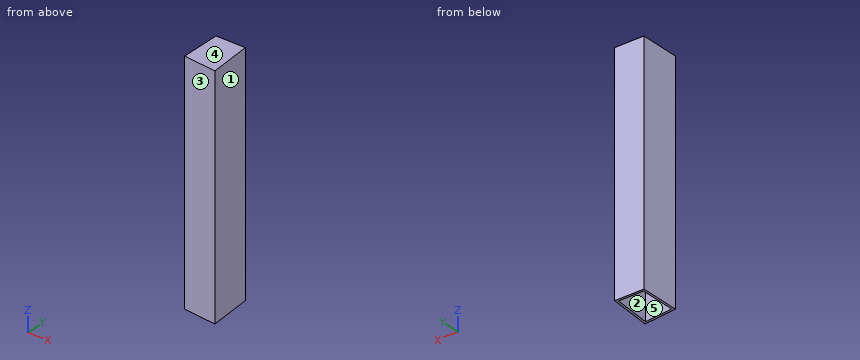
from build123d import *

# Parameters (mm, degrees)
F1_DEPTH = 25.4
F2_DEPTH = 233.172
F3_T     = -2.54


with BuildPart() as f1:
    # F0 (on Top) → F1 (new body)
    with BuildSketch(Plane.XY):
        Polygon((-96.244343, 37.27863), (-129.184976, 37.27863), (-129.184976, -7.511258), (-92.015967, -11.636118), align=None)
    extrude(amount=F1_DEPTH)

    # F0 (on Top) → F2 (join)
    with BuildSketch(Plane.XY):
        Polygon((-96.244343, 37.27863), (-129.184976, 37.27863), (-129.184976, -7.511258), (-92.015967, -11.636118), align=None)
    extrude(amount=-F2_DEPTH)

    # F3
    f3_openings = [f1.faces().sort_by_distance(p)[0] for p in [
        (-111.394879, 13.386796, -233.172),
    ]]
    offset(amount=F3_T, openings=f3_openings)


solid = f1.part
Check sheet for the modelled part. Datum: model origin and axes. Units: mm. Face numbers are marked on the shaded views. A direction names the side the tool comes from. Round coordinates to 2 decimals unless told otherwise and drop trailing zeros. Loops run counter-clockwise (first coordinate to the right, second up) from the corner with the lowest first, then second, coordinate; pieces in that order, holes last.
1. Sectioned sample at C-C on x = -111. Record the boundary of the cut face in (y, z), and give its area (3 significant figures).
2. Mould release check, pull along X, two halves, no side actions. Record for the marked faces 1, 2 and 3: released by +X, released by -X, zero draft, split by the parting line, or undercut.
3. Sectioned sample at A-A on z = -136. Record the boundary of the cut face in (x, y), and give its area (3 significant figures).
4. Set-up check for the marked faces 4 and 5: record each of +Z, -Z, +X, -X, +Y, -Y from which the full face is reachable in a straight line by a thin tool's end or side.
5. Gauge pin test, flat ends, axial feed: pin 1 Ø1.5 at (x, y) = (-122.5, 1) entering from -Z; pin 2 Ø12 at (y, z) = (13, -28) entering from +X; pin 3 Ø5 at (y, z) = (29.5, -94.5) entering from +X. Record the tip position at first contact, or that the pin passes through.
6. Scan lines: probe 1 along Z at (x, y) = (-107.5, 5.5); probe 2 along Y at (x, z) = (-99, -79.5); probe 3 along Y at (x, z) = (-120, -114). Record each from-to range of solid material in increasing order.
7. Sectioned sample at B-B on y = 22. Record the boundary of the cut face in (x, z), and give its area (3 significant figures).
Recorded:
1. outline: (-9.53, -233.17) - (-6.97, -233.17) - (-6.97, 22.86) - (34.74, 22.86) - (34.74, -233.17) - (37.28, -233.17) - (37.28, 25.4) - (-9.53, 25.4) - close
1. area: 1,420 mm2
2. face 1: released by +X
2. face 2: undercut
2. face 3: released by -X
3. outline: (-129.18, -7.51) - (-92.02, -11.64) - (-96.24, 37.28) - (-129.18, 37.28) - close; hole (-126.64, -5.24) - (-94.81, -8.77) - (-98.57, 34.74) - (-126.64, 34.74) - close
3. area: 391 mm2
4. face 4: +Z, +X, -X, +Y, -Y
4. face 5: -Z
5. pin 1: stops at z = 22.86
5. pin 2: stops at x = -93.63
5. pin 3: stops at x = -95.36
6. probe 1: z = 22.86 to 25.4
6. probe 2: y = -10.86 to -8.31, 34.74 to 37.28
6. probe 3: y = -8.53 to -5.97, 34.74 to 37.28
7. outline: (-129.18, -233.17) - (-126.64, -233.17) - (-126.64, 22.86) - (-97.47, 22.86) - (-97.47, -233.17) - (-94.92, -233.17) - (-94.92, 25.4) - (-129.18, 25.4) - close
7. area: 1,390 mm2
